Could you check a few things on this model? Use its own coordinates, in mm. Coordinates: 2 decimals unless noted, no trailing zeros. Loops run counter-clockwise (first coordinate to the right, second up) from the corner with the lowest first, then second, coordinate; pieces in that order, holes last. Notation, with made-up numbers: (47, 50) - (63, 50) arc R24 ccw to (63, 67) - close; hole circle Ø2 at (-28, -8.75). An arc over 180 degrees is marked (long way). Use CSV: the item, a comma, the result in double quotes.
from build123d import *

# Parameters (mm, degrees)
F0_R     = 9.25
F1_DEPTH = 25.4
F3_DEPTH = 12.7


with BuildPart() as f1:
    # F0 (on Front) → F1 (new body)
    with BuildSketch(Plane.XZ):
        with BuildLine():
            Line((-6.943914, 10.433888), (-9.709526, 4.61385))
            ThreePointArc((-9.709526, 4.61385), (0, -10.75), (9.709526, 4.61385))
            Line((9.709526, 4.61385), (6.943914, 10.433888))
            Line((6.943914, 10.433888), (2.587756, 10.433888))
            Line((2.587756, 10.433888), (-2.587756, 10.433888))
            Line((-2.587756, 10.433888), (-6.943914, 10.433888))
        make_face()
        Circle(F0_R, mode=Mode.SUBTRACT)
    extrude(amount=F1_DEPTH)

    # F2 (on Right) → F3 (cut, symmetric)
    with BuildSketch(Plane.YZ):
        with BuildLine():
            ThreePointArc((-12.888511, -10.942341), (-13.328314, 0.984679), (-19.44893, 11.230912))
            Line((-19.44893, 11.230912), (-29.896255, 11.230912))
            Line((-29.896255, 11.230912), (-28.956093, -13.811551))
            Line((-28.956093, -13.811551), (-12.888511, -10.942341))
        make_face()
        with BuildLine():
            Line((6.906466, 11.230912), (-3.540859, 11.230912))
            ThreePointArc((-3.540859, 11.230912), (-9.661475, 0.984679), (-10.101278, -10.942341))
            Line((-10.101278, -10.942341), (5.966304, -13.811551))
            Line((5.966304, -13.811551), (6.906466, 11.230912))
        make_face()
    extrude(amount=F3_DEPTH, both=True, mode=Mode.SUBTRACT)


solid = f1.part
(1) Will these pins go through, and if not, where does the flat tip stop? pin 1 (8 mm diameter, centred on x = 7, z = -8.5, fed in from -Y); pin 2 (6 mm diameter, centred on x = 5.5, y = -17, fed in from -Z); pin 3 (4 mm diameter, centred on x = -8, y = -10, fed in from -Z).
Computed:
pin 1,"stops at y = -12.74"
pin 2,"stops at z = 5.11"
pin 3,"stops at z = -8.88"
(2) Suppose I cut it at D-D (y = -17). Write out the boundary of the cut face in (x, z), plus the area to 3 significant figures.
Computed:
outline,"(-7.92, 8.39) - (-3.9, 8.39) arc R9.25 cw to (3.9, 8.39) - (7.92, 8.39) - (6.94, 10.43) - (-6.94, 10.43) - close"
area,"25.9 mm²"
(3) Please list where these lines run through material, in increasing order: line 1 (X direction, y = -11.75, z = 0); line 2 (Z direction, x = 0, y = -10.75); line 3 (Z direction, x = 0, y = -9).
Computed:
line 1,"x = -10.75 to -9.25, 9.25 to 10.75"
line 2,"z = -10.75 to -9.25, 9.25 to 10.43"
line 3,"z = 9.25 to 10.43"
(4) Suppose I cut it at A-A (x = 0). Write out the boundary of the cut face in (y, z).
Computed:
outline,"(-18.68, 10.43) arc R24.04 cw to (-17.66, 9.25) - (-5.33, 9.25) arc R24.04 cw to (-4.31, 10.43) - close; (-12.85, -10.75) - (-10.14, -10.75) arc R24.04 cw to (-10.41, -9.25) - (-12.58, -9.25) arc R24.04 cw to start"
(5) Suppose I cut it at B-B (z = 0). Write out the boundary of the cut face in (x, y), plus the area to 3 significant figures.
Computed:
outline,"(-10.75, -13.06) - (-9.25, -13.06) - (-9.25, -9.93) - (-10.75, -9.93) - close; (9.25, -13.06) - (10.75, -13.06) - (10.75, -9.93) - (9.25, -9.93) - close"
area,"9.39 mm²"
(6) Thinking about a two-plate mould opening in Z: for faces 1 (the face through (-8, -11.39, 8.21)), 2 (the face through (-1.2, -11.41, 9.17)), 3 (the face through (-0.303, -11.45, -10.746)), which applies, +Z half, -Z half, draft (parallel to the pull), parting line (faces both ways), or undercut?
Computed:
face 1,"+Z half"
face 2,"undercut"
face 3,"parting line"
(7) Suppose I cut it at C-C (y = -9.5). Write out the boundary of the cut face in (x, z), plus the area to 3 significant figures.
Computed:
outline,"(-10.64, 1.51) - (-9.13, 1.51) arc R9.25 cw to (9.13, 1.51) - (10.64, 1.51) arc R10.75 ccw to (9.71, 4.61) - (6.94, 10.43) - (-6.94, 10.43) - (-9.71, 4.61) arc R10.75 ccw to start"
area,"54.0 mm²"
